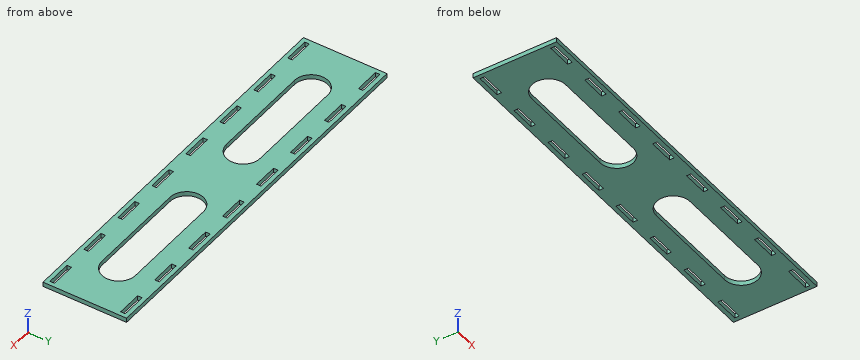
```python
from build123d import *

# Parameters (mm, degrees)
SKETCH1_W           = 460
SKETCH1_H           = 100
SKETCH1_W_2         = 30
SKETCH1_H_2         = 5.4
BOSS_EXTRUDE1_DEPTH = 5.4
CUT_EXTRUDE1_DEPTH  = 6.4


with BuildPart() as part:
    # Sketch1 → Boss-Extrude1 (new body)
    with BuildSketch(Plane.XY):
        with Locations((15.553483591, 15.102805507)):
            Rectangle(SKETCH1_W, SKETCH1_H)
        with Locations((-134.446516409, 57.402805507)):
            Rectangle(SKETCH1_W_2, SKETCH1_H_2, mode=Mode.SUBTRACT)
        with Locations((-194.446516409, 57.402805507)):
            Rectangle(SKETCH1_W_2, SKETCH1_H_2, mode=Mode.SUBTRACT)
        with Locations((-74.446516409, 57.402805507)):
            Rectangle(SKETCH1_W_2, SKETCH1_H_2, mode=Mode.SUBTRACT)
        with Locations((-14.446516409, 57.402805507)):
            Rectangle(SKETCH1_W_2, SKETCH1_H_2, mode=Mode.SUBTRACT)
        with Locations((45.553483591, 57.402805507)):
            Rectangle(SKETCH1_W_2, SKETCH1_H_2, mode=Mode.SUBTRACT)
        with Locations((105.553483591, 57.402805507)):
            Rectangle(SKETCH1_W_2, SKETCH1_H_2, mode=Mode.SUBTRACT)
        with Locations((165.553483591, 57.402805507)):
            Rectangle(SKETCH1_W_2, SKETCH1_H_2, mode=Mode.SUBTRACT)
        with Locations((225.553483591, 57.402805507)):
            Rectangle(SKETCH1_W_2, SKETCH1_H_2, mode=Mode.SUBTRACT)
        with Locations((225.553483591, -27.197194493)):
            Rectangle(SKETCH1_W_2, SKETCH1_H_2, mode=Mode.SUBTRACT)
        with Locations((165.553483591, -27.197194493)):
            Rectangle(SKETCH1_W_2, SKETCH1_H_2, mode=Mode.SUBTRACT)
        with Locations((105.553483591, -27.197194493)):
            Rectangle(SKETCH1_W_2, SKETCH1_H_2, mode=Mode.SUBTRACT)
        with Locations((45.553483591, -27.197194493)):
            Rectangle(SKETCH1_W_2, SKETCH1_H_2, mode=Mode.SUBTRACT)
        with Locations((-14.446516409, -27.197194493)):
            Rectangle(SKETCH1_W_2, SKETCH1_H_2, mode=Mode.SUBTRACT)
        with Locations((-74.446516409, -27.197194493)):
            Rectangle(SKETCH1_W_2, SKETCH1_H_2, mode=Mode.SUBTRACT)
        with Locations((-134.446516409, -27.197194493)):
            Rectangle(SKETCH1_W_2, SKETCH1_H_2, mode=Mode.SUBTRACT)
        with Locations((-194.446516409, -27.197194493)):
            Rectangle(SKETCH1_W_2, SKETCH1_H_2, mode=Mode.SUBTRACT)
    extrude(amount=BOSS_EXTRUDE1_DEPTH)

    # Sketch2 → Cut-Extrude1 (cut, through all)
    with BuildSketch(Plane.XY.offset(5.4)):
        with BuildLine():
            Line((-154.446516409, 35.102805507), (-34.446516409, 35.102805507))
            ThreePointArc((-34.446516409, 35.102805507), (-14.446516409, 15.102805507), (-34.446516409, -4.897194493))
            Line((-34.446516409, -4.897194493), (-154.446516409, -4.897194493))
            ThreePointArc((-154.446516409, -4.897194493), (-174.446516409, 15.102805507), (-154.446516409, 35.102805507))
        make_face()
        with BuildLine():
            Line((65.553483591, -4.897194493), (185.553483591, -4.897194493))
            ThreePointArc((185.553483591, -4.897194493), (205.553483591, 15.102805507), (185.553483591, 35.102805507))
            Line((185.553483591, 35.102805507), (65.553483591, 35.102805507))
            ThreePointArc((65.553483591, 35.102805507), (45.553483591, 15.102805507), (65.553483591, -4.897194493))
        make_face()
    extrude(amount=-CUT_EXTRUDE1_DEPTH, mode=Mode.SUBTRACT)


solid = part.part
```
Geometry: final body of the model. Coordinates: model frame, mm. Round coordinates to 2 decimals unless told otherwise and drop trailing zeros. Order: outer loops, then holes, each group sorted by start corner. A loop starts at its lowest first (then second) coordinate and runs counter-clockwise, first axis right, second up. Notation, with made-up numbers: M 71.5,85.25 L 128.5,85.25 A20 ccw 128.5,117.25 Z; hole C 30.5,31 d3. An arc over 180 degrees is marked long. One line per item, written item: value.
(1) Cut plane C-C (x = -5). Return the cut outline in (y, z).
Result sheet:
outline: M -34.9,0 L -29.9,0 L -29.9,5.4 L -34.9,5.4 Z; M -24.5,0 L 54.7,0 L 54.7,5.4 L -24.5,5.4 Z; M 60.1,0 L 65.1,0 L 65.1,5.4 L 60.1,5.4 Z
(2) Cut plane B-B (x = 84.5). Return the cut outline in (y, z), and give its area (3 significant figures).
Result sheet:
outline: M -34.9,0 L -4.9,0 L -4.9,5.4 L -34.9,5.4 Z; M 35.1,0 L 65.1,0 L 65.1,5.4 L 35.1,5.4 Z
area: 324 mm2
(3) Cut plane A-A (x = -134). Return the cut outline in (y, z), and give its area (3 significant figures).
Result sheet:
outline: M -34.9,0 L -29.9,0 L -29.9,5.4 L -34.9,5.4 Z; M -24.5,0 L -4.9,0 L -4.9,5.4 L -24.5,5.4 Z; M 35.1,0 L 54.7,0 L 54.7,5.4 L 35.1,5.4 Z; M 60.1,0 L 65.1,0 L 65.1,5.4 L 60.1,5.4 Z
area: 266 mm2
(4) Pin query (flat end, axial travel): P1, Ø2, axis at x = 9.5, y = -12.5, coming from the -Z side. Return the tip coordinate at first contact, or that it passes through.
Result sheet:
P1: z = 0
(5) Line query: probe 1 along Y at (x, z) = (-11, 3.1); probe 2 along Y at (x, z) = (-143, 0.4); probe 3 along X at (y, z) = (17, 4.95). Output: solid intervals per line, ascending. Write a range as [from, to].
Result sheet:
probe 1: [-34.9, -29.9], [-24.5, 54.7], [60.1, 65.1]
probe 2: [-34.9, -29.9], [-24.5, -4.9], [35.1, 54.7], [60.1, 65.1]
probe 3: [-214.45, -174.36], [-14.54, 45.64], [205.46, 245.55]
(6) Cut plane D-D (z = 2.15). Give the number of separate pieces and of enclosed holes in the cut face, and give its area (3 significant figures).
Result sheet:
separate pieces: 1
enclosed holes: 18
area: 31,300 mm2
